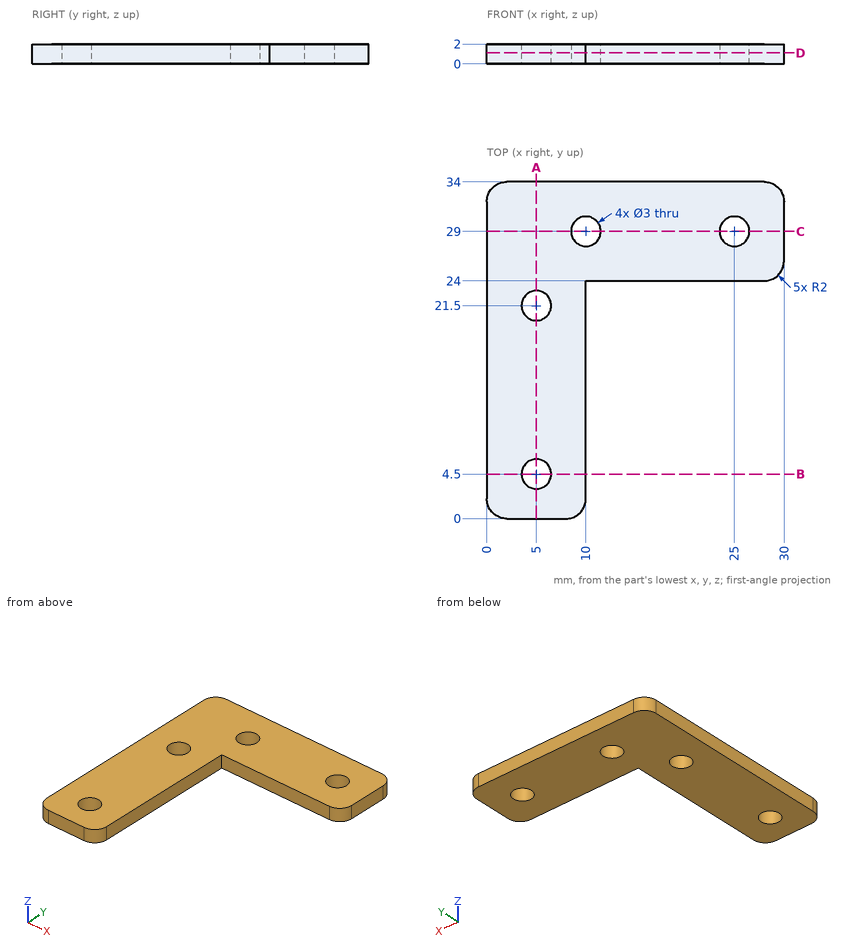
Part print with two shaded views. Sizes in mm from the minimum x, y, z corner. Round coordinates to 2 decimals unless told otherwise and drop trailing zeros. Loops run counter-clockwise (first coordinate to the right, second up) from the corner with the lowest first, then second, coordinate; pieces in that order, holes last. Notation, with made-up numbers: (2, -38.75) - (46, -38.75) arc R20 cw to (46, -30.75) - close; hole circle Ø10 at (52, 88.25). An arc over 180 degrees is marked (long way). Answer as a JSON object with one key per item and string values.
Item 1: Band-saw the part on B-B on y = 4.5. List the corners of the cut face in (x, z).
Output:
{"outline": "(0, 0) - (3.5, 0) - (3.5, 2) - (0, 2) - close; (6.5, 0) - (10, 0) - (10, 2) - (6.5, 2) - close"}
Item 2: Band-saw the part on A-A on x = 5. List the corners of the cut face in (y, z).
Output:
{"outline": "(0, 0) - (3, 0) - (3, 2) - (0, 2) - close; (6, 0) - (20, 0) - (20, 2) - (6, 2) - close; (23, 0) - (34, 0) - (34, 2) - (23, 2) - close"}
Item 3: Band-saw the part on C-C on y = 29. List the corners of the cut face in (x, z), plus the area to 3 significant figures.
Output:
{"outline": "(0, 0) - (8.5, 0) - (8.5, 2) - (0, 2) - close; (11.5, 0) - (23.5, 0) - (23.5, 2) - (11.5, 2) - close; (26.5, 0) - (30, 0) - (30, 2) - (26.5, 2) - close", "area": "48.0 mm2"}
Item 4: Band-saw the part on D-D on z = 1.1. List the corners of the cut face in (x, y).
Output:
{"outline": "(0, 2) arc R2 ccw to (2, 0) - (8, 0) arc R2 ccw to (10, 2) - (10, 24) - (28, 24) arc R2 ccw to (30, 26) - (30, 32) arc R2 ccw to (28, 34) - (2, 34) arc R2 ccw to (0, 32) - close; hole circle Ø3 at (5, 4.5); hole circle Ø3 at (5, 21.5); hole circle Ø3 at (10, 29); hole circle Ø3 at (25, 29)"}
Item 5: Wall check: L1, parallel to Y at x = 5, z = 0.65; L2, parallel to Y at x = 6, z = 0.55; L3, parallel to X at y = 28, z = 1.9. Give the ranges that are in metal, low to high.
Output:
{"L1": "0 to 3, 6 to 20, 23 to 34", "L2": "0 to 3.38, 5.62 to 20.38, 22.62 to 34", "L3": "0 to 8.88, 11.12 to 23.88, 26.12 to 30"}
